Source: CAD feature listing. Evaluate the final solid. Frame: model axes, mm. Round coordinates to 2 decimals unless told otherwise and drop trailing zeros. Write each loop counter-clockwise with the first axis right and the second up, starting at its lowest first coordinate (ties: lowest second). Pieces come first, ordered by that corner, then holes. Notation, with made-up numbers: M 44.5,89 L 69.5,89 A16 ccw 69.5,113 Z; hole C 44.5,-3.75 d4. An arc over 180 degrees is marked long. Use a Markdown table: item, result.
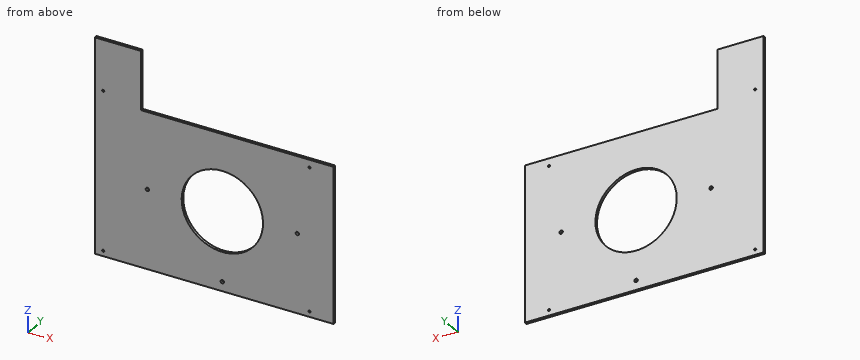
```python
from build123d import *

# Parameters (mm, degrees)
CROQUIS2_R              = 75
CROQUIS2_R_2            = 2
CROQUIS2_R_3            = 3.175
SALIENTE_EXTRUIR2_DEPTH = 5


with BuildPart() as part:
    # Croquis2 → Saliente-Extruir2 (new body)
    with BuildSketch(Plane(origin=(0, 0, 0), x_dir=(1, 0, 0), z_dir=(0, 1, 0))):
        Polygon((-164.024069274, 177.568942162), (-164.024069274, -142.431057838), (-164.024069274, -189.256710106), (-164.024069274, -222.426710106), (-79.024069274, -222.426710106), (-79.024069274, -189.256710106), (-79.024069274, -142.431057838), (-79.024069274, -112.958468136), (275.975930726, -112.958468136), (275.975930726, 177.568942162), align=None)
        with Locations(Location((70.975930726, 30.02579809, 0), (0, 0, 270))):
            Circle(CROQUIS2_R, mode=Mode.SUBTRACT)
        with Locations(Location((-148.613055051, 167.568942162, 0), (0, 0, 270))):
            Circle(CROQUIS2_R_2, mode=Mode.SUBTRACT)
        with Locations(Location((-148.613055051, -128.145081947, 0), (0, 0, 270))):
            Circle(CROQUIS2_R_2, mode=Mode.SUBTRACT)
        with Locations(Location((231.386944949, -98.672492245, 0), (0, 0, 270))):
            Circle(CROQUIS2_R_2, mode=Mode.SUBTRACT)
        with Locations(Location((231.386944949, 167.568942162, 0), (0, 0, 270))):
            Circle(CROQUIS2_R_2, mode=Mode.SUBTRACT)
        with Locations(Location((209.175930726, 30.02579809, 0), (0, 0, 270))):
            Circle(CROQUIS2_R_3, mode=Mode.SUBTRACT)
        with Locations(Location((-67.224069274, 30.02579809, 0), (0, 0, 270))):
            Circle(CROQUIS2_R_3, mode=Mode.SUBTRACT)
        with Locations(Location((70.975930726, 160.02579809, 0), (0, 0, 270))):
            Circle(CROQUIS2_R_3, mode=Mode.SUBTRACT)
    extrude(amount=SALIENTE_EXTRUIR2_DEPTH)


solid = part.part
```
Q1. Section B-B on y = 1.4. Give the number of separate pieces and of enclosed holes in the cut face, plus the area to 3 significant figures.
Results are:
| item | result |
|---|---|
| separate pieces | 1 |
| enclosed holes | 8 |
| area | 119,000 mm^2 |
Q2. First-contact query: pin 1 Ø6 at (x, z) = (139.5, 118.5) entering from +Y; pin 2 Ø2.5 at (y, z) = (2.5, 155) entering from +X; pin 3 Ø6 at (x, z) = (93, -115.5) entering from -Y; pin 4 Ø1.5 at (x, y) = (64.5, 1.5) entering from +Z. Flat tips, straight axial feed; report the tip coordinate or a pass-through.
Results are:
| item | result |
|---|---|
| pin 1 | through |
| pin 2 | x = -79.02 |
| pin 3 | y = 0 |
| pin 4 | z = 112.96 |
Q3. Section A-A on x = 26.5. Return loops of the section in (y, z).
Results are:
| item | result |
|---|---|
| outline | M 0,-177.57 L 5,-177.57 L 5,-90.42 L 0,-90.42 Z; M 0,30.36 L 5,30.36 L 5,112.96 L 0,112.96 Z |
Q4. Section C-C on z = -0.5. Return loops of the section in (x, y), plus the area to 3 significant figures.
Results are:
| item | result |
|---|---|
| outline | M -164.02,0 L 2.03,0 L 2.03,5 L -164.02,5 Z; M 139.92,0 L 275.98,0 L 275.98,5 L 139.92,5 Z |
| area | 1,510 mm^2 |
Q5. Line query: L1, parallel to Z at x = 209, y = 1.15; L2, parallel to X at y = 2.75, z = 128; L3, parallel to Z at x = 164, y = 3.4. Output: solid intervals per line, ascending.
Results are:
| item | result |
|---|---|
| L1 | -177.57 to -33.2, -26.86 to 112.96 |
| L2 | -164.02 to -150.61, -146.62 to -79.02 |
| L3 | -177.57 to 112.96 |
Q6. Section D-D on x = 242.5. Return loops of the section in (y, z).
Results are:
| item | result |
|---|---|
| outline | M 0,-177.57 L 5,-177.57 L 5,112.96 L 0,112.96 Z |
